The listing builds one solid part. Answer for the finished solid, in the listing's coordinates (mm). Round coordinates to 2 decimals unless told otherwise and drop trailing zeros. Write each loop counter-clockwise with the first axis right and the second up, starting at its lowest first coordinate (ties: lowest second). Pieces come first, ordered by that corner, then holes. Notation, with made-up numbers: M 3.5,76 L 12.5,76 A9 cw 12.5,92 Z; hole C -27,-14.75 d7. An arc over 180 degrees is marked long. Write each question's results on one line, items separated by ' | '.
from build123d import *

# Parameters (mm, degrees)
BOSS_EXTRUDE1_DEPTH = 2.5654
SKETCH7_R           = 4.6863
CUT_EXTRUDE1_DEPTH  = 9.857267478
FILLET1_SIZE        = 0.508
FILLET2_SIZE        = 0.508


with BuildPart() as part:
    # Sketch4 → Boss-Extrude1 (new body)
    with BuildSketch(Plane(origin=(0, 0, 0), x_dir=(1, 0, 0), z_dir=(0, 1, 0))):
        Polygon((6.408472518, 0), (3.204236259, 5.5499), (-3.204236259, 5.5499), (-6.408472518, 0), (-3.204236259, -5.5499), (3.204236259, -5.5499), align=None)
    extrude(amount=BOSS_EXTRUDE1_DEPTH)

    # Sketch7 → Cut-Extrude1 (cut, through all)
    with BuildSketch(Plane(origin=(0, 2.5654, 0), x_dir=(1, 0, 0), z_dir=(0, 1, 0))):
        with Locations(Location((0, 0, 0), (0, 0, 270))):
            Circle(SKETCH7_R)
    extrude(amount=-CUT_EXTRUDE1_DEPTH, mode=Mode.SUBTRACT)

    # Fillet1
    fillet1_edges = [part.edges().sort_by_distance(p)[0] for p in [
        (0, 2.5654, -4.6863),
    ]]
    chamfer(fillet1_edges, length=FILLET1_SIZE)

    # Fillet2
    fillet2_edges = [part.edges().sort_by_distance(p)[0] for p in [
        (0, 0, -4.6863),
    ]]
    chamfer(fillet2_edges, length=FILLET2_SIZE)


solid = part.part
1) Section B-B (x = 0) is taken. Determine the outline of the cut face in (y, z), then the cut area to 3 significant figures.
Return value:
outline: M 0,-5.55 L 2.57,-5.55 L 2.57,-5.19 L 2.06,-4.69 L 0.51,-4.69 L 0,-5.19 Z; M 0,5.19 L 0.51,4.69 L 2.06,4.69 L 2.57,5.19 L 2.57,5.55 L 0,5.55 Z | area: 3.91 mm²
2) Section A-A (y = 1.65) is taken. Determine the outline of the cut face in (x, z), then the cut area to 3 significant figures.
Return value:
outline: M -6.41,0 L -3.2,-5.55 L 3.2,-5.55 L 6.41,0 L 3.2,5.55 L -3.2,5.55 Z; hole C 0,0 d9.37 | area: 37.7 mm²
3) Find the intervals of material crossed by line 1 (X direction, y = 1.85, z = -1.75); line 2 (Z direction, x = -0.75, y = 2.25); line 3 (Z direction, x = -1.75, y = 1.25), in increasing order.
Return value:
line 1: -5.4 to -4.35, 4.35 to 5.4 | line 2: -5.55 to -4.82, 4.82 to 5.55 | line 3: -5.55 to -4.35, 4.35 to 5.55
4) Each of these flat-tipped pins is pushed along its axis until it touches: pin 1 (5.5 mm diameter, centred on x = 0, z = 0, fed in from +Y); pin 2 (1.5 mm diameter, centred on y = 0.5, z = 3.5, fed in from -X); pin 3 (1.5 mm diameter, centred on y = 1.5, z = 2, fed in from +X); pin 4 (1 mm diameter, centred on y = 0.5, z = -4, fed in from +X). Where does it stop, or does it pass through?
Return value:
pin 1: through | pin 2: x = -4.82 | pin 3: x = 5.69 | pin 4: x = 4.39
5) The mould has two halves that part along X. Classify faces 1 (the face through (5, 2.565, 2)), 2 (the face through (1.41, 1.29, 4.47)), 3 (the face through (-4.784, 1.265, -2.814)): +X half, -X half, draft (parallel to the pull), parting line (faces both ways), or undercut.
Return value:
face 1: draft | face 2: undercut | face 3: -X half
6) Section C-C (y = 0.25) is taken. Determine the outline of the cut face in (x, z).
Return value:
outline: M -6.41,0 L -3.2,-5.55 L 3.2,-5.55 L 6.41,0 L 3.2,5.55 L -3.2,5.55 Z; hole C 0,0 d9.89
